from build123d import *

# Parameters (mm, degrees)
F0_W     = 180
F0_H     = 20
F1_DEPTH = 20
F3_DEPTH = 25
F4_R     = 2
F5_W     = 100
F5_H     = 16
F6_DEPTH = 3


with BuildPart() as f1:
    # F0 (on Front) → F1 (new body)
    with BuildSketch(Plane.XZ):
        with Locations((90, 10)):
            Rectangle(F0_W, F0_H)
    extrude(amount=-F1_DEPTH)

    # F2 (on face) → F3 (cut)
    with BuildSketch(Plane.XZ):
        with BuildLine():
            Line((75.7071421427, 20), (4.2928578573, 20))
            ThreePointArc((4.2928578573, 20), (20.635083269, 8.9022777135), (40, 5))
            ThreePointArc((40, 5), (59.364916731, 8.9022777135), (75.7071421427, 20))
        make_face()
        with BuildLine():
            Line((175.7071421427, 20), (104.2928578573, 20))
            ThreePointArc((104.2928578573, 20), (120.635083269, 8.9022777135), (140, 5))
            ThreePointArc((140, 5), (159.364916731, 8.9022777135), (175.7071421427, 20))
        make_face()
        with BuildLine():
            Line((104.2928578573, 20), (75.7071421427, 20))
            ThreePointArc((75.7071421427, 20), (59.364916731, 8.9022777135), (40, 5))
            Line((40, 5), (140, 5))
            ThreePointArc((140, 5), (120.635083269, 8.9022777135), (104.2928578573, 20))
        make_face()
    extrude(amount=-F3_DEPTH, mode=Mode.SUBTRACT)

    # F4
    f4_edges = [f1.edges().sort_by_distance(p)[0] for p in [
        (0, 10, 20),
        (4.292858, 10, 20),
        (175.707142, 10, 20),
        (180, 10, 20),
    ]]
    fillet(f4_edges, radius=F4_R)

    # F5 (on face) → F6 (cut)
    with BuildSketch(Plane.XY.offset(5)):
        with Locations((90, 10)):
            Rectangle(F5_W, F5_H)
    extrude(amount=-F6_DEPTH, mode=Mode.SUBTRACT)


solid = f1.part
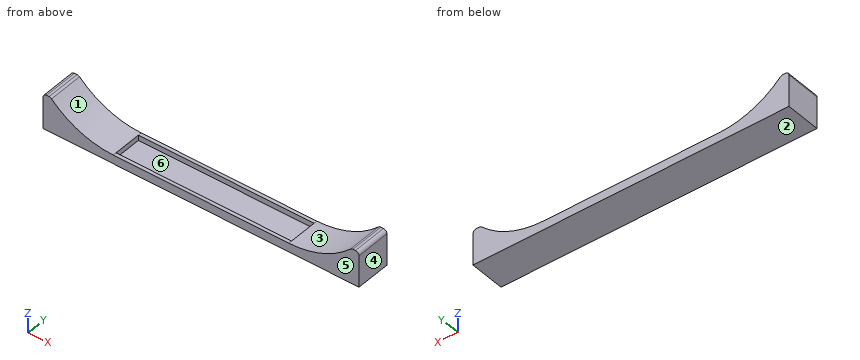
Design review of the part built by this model. Coordinates are the model's own, in mm. Face numbers are marked on the shaded views. A direction names the side the tool comes from. Coordinates: 2 decimals unless noted, no trailing zeros. Order: outer loops, then holes, each group sorted by start corner. A loop starts at its lowest first (then second) coordinate and runs counter-clockwise, first axis right, second up. Notation, with made-up numbers: (-39.75, 39.5) -> (-20.75, 39.5) arc R21 cw to (-20.75, 71.5) -> close; hole circle Ø2 at (76.5, 81.25). An arc over 180 degrees is marked (long way). One line per item, written item: value.
1) Draft analysis for pull direction X (two halves, no side actions). For the marked faces 1, 2, 3 and 4, state which applies: +X half, -X half, draft (parallel to the pull), parting line (faces both ways), or undercut.
Output values:
face 1: undercut
face 2: draft
face 3: undercut
face 4: +X half
2) Machinability: for the marked faces 5 and 6, which of the approach directions +Z, -Z, +X, -X, +Y, -Y give a long, thin tool a straight path to every point of the face, cutting with its end or side? Answer none if there is none.
Output values:
face 5: +Z, -Z, +X, -X, -Y
face 6: +Z
3) We need section C-C, the plane z = 13.5. Give the boundary of the cut face in (x, y).
Output values:
outline: (0, 0) -> (12.11, 0) -> (12.11, 20) -> (0, 20) -> close; (167.89, 0) -> (180, 0) -> (180, 20) -> (167.89, 20) -> close
4) We need section A-A, the plane y = 6. Give the boundary of the cut face in (x, z).
Output values:
outline: (0, 0) -> (180, 0) -> (180, 18) arc R2 ccw to (178, 20) -> (176.54, 20) arc R2 ccw to (175.13, 19.42) arc R50 cw to (140, 5) -> (140, 2) -> (40, 2) -> (40, 5) arc R50 cw to (4.87, 19.42) arc R2 ccw to (3.46, 20) -> (2, 20) arc R2 ccw to (0, 18) -> close
5) Clearance check with flat-ended pins moving along their axes: P1, Ø10, axis at x = 61, y = 14, coming from the +Z side; P2, Ø1.5, axis at x = 123, y = 10.5, coming from the +Z side. State where each tip first meets the part, or that it passes through.
Output values:
P1: stops at z = 5
P2: stops at z = 2
6) To check wall thickness, follow probe 1 along Y at (x, z) = (59.5, 4); probe 2 along Z at (x, y) = (59, 13); probe 3 along X at (y, z) = (7.25, 3.75). State the ranges of each line that lie inside material, in increasing order. Write a range as [from, to].
Output values:
probe 1: y = [0, 2], [18, 20]
probe 2: z = [0, 2]
probe 3: x = [0, 40], [140, 180]
7) We need section B-B, the plane x = 82.5. Give the boundary of the cut face in (y, z).
Output values:
outline: (0, 0) -> (20, 0) -> (20, 5) -> (18, 5) -> (18, 2) -> (2, 2) -> (2, 5) -> (0, 5) -> close
8) We need section D-D, the plane x = 30.5. Give the boundary of the cut face in (y, z), then the cut area to 3 significant figures.
Output values:
outline: (0, 0) -> (20, 0) -> (20, 5.91) -> (0, 5.91) -> close
area: 118 mm2
